Could you check a few things on this model? Use its own coordinates, in mm. A direction names the side the tool comes from. Coordinates: 2 decimals unless noted, no trailing zeros. Loops run counter-clockwise (first coordinate to the right, second up) from the corner with the lowest first, then second, coordinate; pieces in that order, holes last. Notation, with made-up numbers: M 37.25,47 L 84.25,47 A12 ccw 84.25,68 Z; hole C -18,34.25 d6. An arc over 180 degrees is marked long. Write each question's results on one line, items separated by ' | '.
```python
from build123d import *

# Parameters (mm, degrees)
SKETCH1_R           = 24.5
SKETCH1_R_2         = 16
BOSS_EXTRUDE1_DEPTH = 3
SKETCH2_R           = 24.5
BOSS_EXTRUDE2_DEPTH = 5
SKETCH3_R           = 2.05
CUT_EXTRUDE1_DEPTH  = 36.559808773
SKETCH4_R           = 1.5
CUT_EXTRUDE2_DEPTH  = 3


with BuildPart() as part:
    # Sketch1 → Boss-Extrude1 (new body)
    with BuildSketch(Plane.XY):
        Circle(SKETCH1_R)
        Circle(SKETCH1_R_2, mode=Mode.SUBTRACT)
    extrude(amount=BOSS_EXTRUDE1_DEPTH)

    # Sketch2 → Boss-Extrude2 (add)
    with BuildSketch(Plane.XY.offset(3)):
        Circle(SKETCH2_R)
    extrude(amount=BOSS_EXTRUDE2_DEPTH)

    # Sketch3 → Cut-Extrude1 (cut, through all)
    with BuildSketch(Plane(origin=(0, 0, 0), x_dir=(-1, 0, 0), z_dir=(0, 0, -1))):
        with Locations((0, 20.25)):
            Circle(SKETCH3_R)
        with Locations((20.25, 0)):
            Circle(SKETCH3_R)
        with Locations((0, -20.25)):
            Circle(SKETCH3_R)
        with Locations((-20.25, 0)):
            Circle(SKETCH3_R)
    extrude(amount=-CUT_EXTRUDE1_DEPTH, mode=Mode.SUBTRACT)

    # Sketch4 → Cut-Extrude2 (cut)
    with BuildSketch(Plane(origin=(0, 0, 3), x_dir=(-1, 0, 0), z_dir=(0, 0, -1))):
        Circle(SKETCH4_R)
    extrude(amount=-CUT_EXTRUDE2_DEPTH, mode=Mode.SUBTRACT)


solid = part.part
```
(1) If we mould it in two halves opening along Y, with no side actions, what happens to faces 3 (the cylindrical face through (22.3, 0.09, 3.94)), 4 (the cylindrical face through (13.17, 20.66, 3.94)), 5 (the flat face through (16, -5, 0))? For each: released by +Y, released by -Y, zero draft, split by the parting line, or undercut.
Reported:
face 3: undercut | face 4: split by the parting line | face 5: zero draft
(2) Will these pins go through, and if not, where does the flat tip stop? P1, Ø4, axis at x = -11, z = 2.5, coming from the +Y side; P2, Ø3.5, axis at x = 0, y = 20.25, coming from the -Z side; P3, Ø12, axis at x = -9.5, y = 7.5, coming from the -Z side; P4, Ø2, axis at x = -1.5, z = 7, coming from the -Y side.
Reported:
P1: stops at y = 22.79 | P2: passes through | P3: stops at z = 0 | P4: stops at y = -24.49
(3) Please list where these lines run through material, in increasing order: probe 1 along Y at (x, z) = (0, 2.4); probe 2 along Y at (x, z) = (0, 5.25); probe 3 along Y at (x, z) = (-2.5, 2). Write a range as from..to.
Reported:
probe 1: y = -24.5..-22.3, -18.2..-16, 16..18.2, 22.3..24.5 | probe 2: y = -24.5..-22.3, -18.2..-1.5, 1.5..18.2, 22.3..24.5 | probe 3: y = -24.37..-15.8, 15.8..24.37
(4) Imagine slicing it at B-B, the plane x = 0. List the corners of the cut face in (y, z) for me.
Reported:
outline: M -24.5,0 L -22.3,0 L -22.3,8 L -24.5,8 Z; M -18.2,0 L -16,0 L -16,3 L -1.5,3 L -1.5,6 L 1.5,6 L 1.5,3 L 16,3 L 16,0 L 18.2,0 L 18.2,8 L -18.2,8 Z; M 22.3,0 L 24.5,0 L 24.5,8 L 22.3,8 Z
(5) Which directions (+Z, -Z, +X, -X, +Y, -Y) give clear straight access to the entire face, cutting with the end or side of a thin tool? Please do faces 1 (the cylindrical face through (1.511, -18.865, 3.944)), 2 (the cylindrical face through (-3.47, -15.62, 1.48)).
Reported:
face 1: +Z, -Z | face 2: -Z
(6) Imagine slicing it at A-A, the plane z = 2. List the corners of the cut face in (x, y) for me.
Reported:
outline: C 0,0 d49; hole C -20.25,0 d4.1; hole C 0,0 d32; hole C 0,-20.25 d4.1; hole C 0,20.25 d4.1; hole C 20.25,0 d4.1
(7) Imagine slicing it at D-D, the plane y = -20.25. List the corners of the cut face in (x, z) for me, and give its area (3 significant figures).
Reported:
outline: M -13.79,0 L -2.05,0 L -2.05,8 L -13.79,8 Z; M 2.05,0 L 13.79,0 L 13.79,8 L 2.05,8 Z | area: 188 mm2
